Check sheet for the modelled part. Datum: model origin and axes. Units: mm. A direction names the side the tool comes from. Round coordinates to 2 decimals unless told otherwise and drop trailing zeros. Write each loop counter-clockwise with the first axis right and the second up, starting at its lowest first coordinate (ties: lowest second). Pieces come first, ordered by that corner, then holes. Notation, with made-up numbers: M 79.25,-8 L 121.25,-8 A24 cw 121.25,22 Z; hole C -23,17.5 d11. An arc over 180 degrees is marked long. Put each result on its own line as item: value.
```python
from build123d import *

# Parameters (mm, degrees)
SKETCH1_W            = 42
SKETCH1_H            = 8
SKETCH1_W_2          = 41
SKETCH1_H_2          = 4.5
BOSS_EXTRUDE1_DEPTH  = 54
CUT_EXTRUDE1_REACH   = 60.078
MIRROR2_COPY_1_REACH = 60.078
FILLET1_R            = 1.8
CUT_EXTRUDE2_START   = -2
SKETCH3_OUTSIDE_W    = 57.776
SKETCH3_OUTSIDE_H    = 23.776
SKETCH3_OUTSIDE_W_2  = 42
SKETCH3_OUTSIDE_H_2  = 5.3
CUT_EXTRUDE2_DEPTH   = 50
CHAMFER1_SIZE        = 1.35


with BuildPart() as part:
    # Sketch1 → Boss-Extrude1 (new body)
    with BuildSketch(Plane.XY):
        Rectangle(SKETCH1_W, SKETCH1_H)
        Rectangle(SKETCH1_W_2, SKETCH1_H_2, mode=Mode.SUBTRACT)
    extrude(amount=BOSS_EXTRUDE1_DEPTH)

    # Sketch2 → Cut-Extrude1 (cut, up to next)
    with BuildSketch(Plane.XY.offset(54), mode=Mode.PRIVATE) as cut_extrude1_sk1:
        Polygon((-16, 4), (-21, 2.302178038), (-21, 4), align=None)
    cut_extrude1_tool1 = extrude(cut_extrude1_sk1.sketch, amount=-CUT_EXTRUDE1_REACH, mode=Mode.PRIVATE) & part.part
    cut_extrude1 = cut_extrude1_tool1.solids().sort_by_distance((-19.333333, 3.434059, 54))[0]
    add(cut_extrude1, mode=Mode.SUBTRACT)

    # Mirror1: Cut-Extrude1 across plane
    add(cut_extrude1.mirror(Plane.ZX), mode=Mode.SUBTRACT)

    # Mirror2: Cut-Extrude1 across plane
    add(cut_extrude1.mirror(Plane(origin=(0, 0, 0), x_dir=(0, 0, 1), z_dir=(1, 0, 0))), mode=Mode.SUBTRACT)

    # Mirror2 copy 1 sketch → Mirror2 copy 1 (cut, up to next)
    with BuildSketch(Plane(origin=(0, 0, 54), x_dir=(-1, 0, 0), z_dir=(0, 0, 1)), mode=Mode.PRIVATE) as mirror2_copy_1_sk1:
        Polygon((-16, 4), (-21, 2.302178038), (-21, 4), align=None)
    mirror2_copy_1_tool1 = extrude(mirror2_copy_1_sk1.sketch, amount=-MIRROR2_COPY_1_REACH, mode=Mode.PRIVATE) & part.part
    add(mirror2_copy_1_tool1.solids().sort_by_distance((19.333333, -3.434059, 54))[0], mode=Mode.SUBTRACT)

    # Fillet1
    fillet1_edges = [part.edges().sort_by_distance(p)[0] for p in [
        (-20.5, 2.25, 27),
        (-20.5, -2.25, 27),
        (20.5, -2.25, 27),
        (20.5, 2.25, 27),
    ]]
    fillet(fillet1_edges, radius=FILLET1_R)

    # Sketch3 outside → Cut-Extrude2 (cut)
    with BuildSketch(Plane.XY.offset(54).offset(CUT_EXTRUDE2_START)):
        Rectangle(SKETCH3_OUTSIDE_W, SKETCH3_OUTSIDE_H)
        Rectangle(SKETCH3_OUTSIDE_W_2, SKETCH3_OUTSIDE_H_2, mode=Mode.SUBTRACT)
    extrude(amount=-CUT_EXTRUDE2_DEPTH, mode=Mode.SUBTRACT)

    # Chamfer1
    chamfer1_edges = [part.edges().sort_by_distance(p)[0] for p in [
        (0, -2.65, 2),
        (0, -2.65, 52),
        (0, 2.65, 52),
        (0, 2.65, 2),
    ]]
    chamfer(chamfer1_edges, length=CHAMFER1_SIZE - 0.0001)  # a hair under: the kernel refuses the full size


solid = part.part
```
1. Access from +Z, -Z, +X, -X, +Y, -Y to the whole of each face (thin tool, end or side, straight path). Record for faces 4 (the flat face through (0, 2.25, 27)), 5 (the flat face through (0, 3, 3)), 6 (the flat face through (0, -3, 51)).
Computed values:
face 4: +Z, -Z
face 5: +X, -X, +Y
face 6: +X, -X, -Y
2. Cross-section at D-D (x = -18). Enter the section's corners in (y, z), then the cut area to 3 significant figures.
Computed values:
outline: M -3.32,0 L -2.25,0 L -2.25,54 L -3.32,54 L -3.32,51.32 L -2.65,50.65 L -2.65,3.35 L -3.32,2.68 Z; M 2.25,0 L 3.32,0 L 3.32,2.68 L 2.65,3.35 L 2.65,50.65 L 3.32,51.32 L 3.32,54 L 2.25,54 Z
area: 51.3 mm2
3. Cross-section at C-C (y = -1.25). Enter the section's corners in (x, z), then the cut area to 3 significant figures.
Computed values:
outline: M -21,0 L -20.31,0 L -20.31,54 L -21,54 Z; M 20.31,0 L 21,0 L 21,54 L 20.31,54 Z
area: 74.3 mm2
4. Scan lines: probe 1 along Y at (x, z) = (11, 50); probe 2 along X at (y, z) = (0.5, 9.5). Record each from-to range of solid material in increasing order.
Computed values:
probe 1: y = -2.65 to -2.25, 2.25 to 2.65
probe 2: x = -21 to -20.5, 20.5 to 21
5. Depth check by flat-ended pin: pin 1 Ø1.5 at (x, z) = (6, 32) entering from +Y; pin 2 Ø1 at (x, z) = (-5.5, 48.5) entering from -Y. Enter the tip coordinate at first touch or a pass-through.
Computed values:
pin 1: stops at y = 2.65
pin 2: stops at y = -2.65
6. Cross-section at B-B (z = 47.5). Enter the section's corners in (x, y), then the cut area to 3 significant figures.
Computed values:
outline: M -21,-2.3 L -19.98,-2.65 L 19.98,-2.65 L 21,-2.3 L 21,2.3 L 19.98,2.65 L -19.98,2.65 L -21,2.3 Z; hole M -20.5,-0.45 A1.8 ccw -18.7,-2.25 L 18.7,-2.25 A1.8 ccw 20.5,-0.45 L 20.5,0.45 A1.8 ccw 18.7,2.25 L -18.7,2.25 A1.8 ccw -20.5,0.45 Z
area: 40.2 mm2
7. Release check for a two-part mould opening along X. For faces 1 (the cylindrical face through (19.987, 1.709, 27.378)), 2 (the flat face through (0, -4, 1)), 3 (the flat face through (-21, 0, 27)) record: +X half, -X half, draft (parallel to the pull), parting line (faces both ways), or undercut.
Computed values:
face 1: undercut
face 2: draft
face 3: -X half
